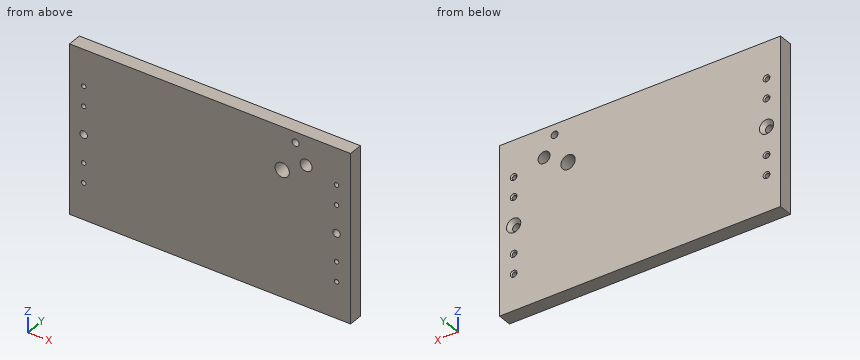
```python
from build123d import *

# Parameters (mm, degrees)
SKETCH1_W                                        = 254
SKETCH1_H                                        = 152.4
BOSS_EXTRUDE1_DEPTH                              = 12.7
SKETCH2_W                                        = 203.2
SKETCH2_H                                        = 63.5
CUT_EXTRUDE1_DEPTH                               = 149.649688866
SKETCH11_W                                       = 203.2
SKETCH11_H                                       = 63.5
BOSS_EXTRUDE2_DEPTH                              = 12.7
SKETCH13_R                                       = 5.3578125
SKETCH13_R_2                                     = 6.4897
CUT_EXTRUDE8_DEPTH                               = 149.649688866
SKETCH14_R                                       = 3.1623
CUT_EXTRUDE9_DEPTH                               = 149.649688866
F_10_32_TAPPED_HOLE2_D                           = 4.0386
F_10_32_TAPPED_HOLE2_CSINK_D                     = 6.096
F_10_32_TAPPED_HOLE2_CSINK_ANGLE                 = 90
MIRROR2_COPY_1_D                                 = 4.0386
MIRROR2_COPY_1_CSINK_D                           = 6.096
MIRROR2_COPY_1_CSINK_ANGLE                       = 90
CSK_FOR_1_4_FLAT_HEAD_MACHINE_SCREW1_D           = 6.7564
CSK_FOR_1_4_FLAT_HEAD_MACHINE_SCREW1_CSINK_D     = 12.8778
CSK_FOR_1_4_FLAT_HEAD_MACHINE_SCREW1_CSINK_ANGLE = 82


with BuildPart() as part:
    # Sketch1 → Boss-Extrude1 (new body)
    with BuildSketch(Plane(origin=(0, 0, 0), x_dir=(1, 0, 0), z_dir=(0, 1, 0))):
        Rectangle(SKETCH1_W, SKETCH1_H)
    extrude(amount=BOSS_EXTRUDE1_DEPTH)

    # Sketch2 → Cut-Extrude1 (cut, through all)
    with BuildSketch(Plane(origin=(0, 12.7, 0), x_dir=(1, 0, 0), z_dir=(0, 1, 0))):
        with Locations((0, -44.45)):
            Rectangle(SKETCH2_W, SKETCH2_H)
        with Locations((0, 44.45)):
            Rectangle(SKETCH2_W, SKETCH2_H)
    extrude(amount=-CUT_EXTRUDE1_DEPTH, mode=Mode.SUBTRACT)

    # Sketch11 → Boss-Extrude2 (add)
    with BuildSketch(Plane(origin=(0, 12.7, 0), x_dir=(1, 0, 0), z_dir=(0, 1, 0))):
        with Locations((0, 44.45)):
            Rectangle(SKETCH11_W, SKETCH11_H)
        with Locations((0, -44.45)):
            Rectangle(SKETCH11_W, SKETCH11_H)
    extrude(amount=-BOSS_EXTRUDE2_DEPTH)

    # Sketch13 → Cut-Extrude8 (cut, through all)
    with BuildSketch(Plane(origin=(0, 12.7, 0), x_dir=(1, 0, 0), z_dir=(0, 1, 0))):
        with Locations(Location((86.819046868, -50.12500008, 0), (0, 0, 270))):
            Circle(SKETCH13_R)
        with Locations(Location((65.16841174, -37.625000061, 0), (0, 0, 270))):
            Circle(SKETCH13_R_2)
    extrude(amount=-CUT_EXTRUDE8_DEPTH, mode=Mode.SUBTRACT)

    # Sketch14 → Cut-Extrude9 (cut, through all)
    with BuildSketch(Plane(origin=(0, 12.7, 0), x_dir=(1, 0, 0), z_dir=(0, 1, 0))):
        with Locations(Location((77.237896866, -66.720038678, 0), (0, 0, 270))):
            Circle(SKETCH14_R)
    extrude(amount=-CUT_EXTRUDE9_DEPTH, mode=Mode.SUBTRACT)

    # #10-32 Tapped Hole2 (through all)
    with Locations(Plane(origin=(0, 12.7, 0), x_dir=(1, 0, 0), z_dir=(0, 1, 0))):
        with Locations((-114.3, -25.3365), (-114.3, -43.2435)):
            f_10_32_tapped_hole2 = CounterSinkHole(F_10_32_TAPPED_HOLE2_D / 2, F_10_32_TAPPED_HOLE2_CSINK_D / 2, counter_sink_angle=F_10_32_TAPPED_HOLE2_CSINK_ANGLE)

    # Mirror1: #10-32 Tapped Hole2 across plane
    add(f_10_32_tapped_hole2.mirror(Plane.XY), mode=Mode.SUBTRACT)

    # Mirror2: #10-32 Tapped Hole2 across plane
    add(f_10_32_tapped_hole2.mirror(Plane(origin=(0, 0, 0), x_dir=(0, 0, 1), z_dir=(1, 0, 0))), mode=Mode.SUBTRACT)

    # Mirror2 copy 1 (through all)
    with Locations(Plane(origin=(0, 12.7, 0), x_dir=(-1, 0, 0), z_dir=(0, 1, 0))):
        with Locations((-114.3, -25.3365), (-114.3, -43.2435)):
            CounterSinkHole(MIRROR2_COPY_1_D / 2, MIRROR2_COPY_1_CSINK_D / 2, counter_sink_angle=MIRROR2_COPY_1_CSINK_ANGLE)

    # CSK for 1/4 Flat Head Machine Screw1 (through all)
    with Locations(Plane(origin=(0, 12.7, 0), x_dir=(1, 0, 0), z_dir=(0, 1, 0))):
        with Locations((-114.3, 0)):
            csk_for_1_4_flat_head_machine_screw1 = CounterSinkHole(CSK_FOR_1_4_FLAT_HEAD_MACHINE_SCREW1_D / 2, CSK_FOR_1_4_FLAT_HEAD_MACHINE_SCREW1_CSINK_D / 2, counter_sink_angle=CSK_FOR_1_4_FLAT_HEAD_MACHINE_SCREW1_CSINK_ANGLE)

    # Mirror3: CSK for 1/4 Flat Head Machine Screw1 across plane
    add(csk_for_1_4_flat_head_machine_screw1.mirror(Plane(origin=(0, 0, 0), x_dir=(0, 0, 1), z_dir=(1, 0, 0))), mode=Mode.SUBTRACT)


solid = part.part
```
CAD build for the part. Positions are in the model's coordinates, mm. Give positions to 0.01 mm unless a question says otherwise; leave off trailing zeros. Write each loop counter-clockwise with the first axis right and the second up, starting at its lowest first coordinate (ties: lowest second). Pieces come first, ordered by that corner, then holes. Notation, with made-up numbers: M 27.5,-5 L 76.5,-5 A14 cw 76.5,21 Z; hole C -37.75,54.5 d8. An arc over 180 degrees is marked long. Return JSON: item names as keys, results as strings. Group by question number.
(1) Drill centre lines: L1, parallel to X at y = 3.25, z = -1.5; L2, parallel to X at y = 0.75, z = -25.5; L3, parallel to Z at x = -114.3, y = 6. Where is each one in solid material? Low to high. Write a range as [from, to].
(2) Band-saw the part on A-A (z = 0). Give the cut face in (x, y).
(3) Flat gauge pins, fed straight in: pin 1 Ø5.5 at (x, z) = (-114.3, 43.24) entering from +Y; pin 2 Ø3.5 at (x, z) = (114.3, -25.34) entering from +Y; pin 3 Ø8 at (x, z) = (114.3, 0) entering from +Y. Where does each tip first touch, or does it go through?
Entries:
{
 "1": {"L1": "x = [-127, -117.33], [-111.27, 111.27], [117.33, 127]", "L2": "x = [-127, -116.31], [-112.29, 112.29], [116.31, 127]", "L3": "z = [-76.2, -45.26], [-41.22, -27.36], [-23.32, -3.38], [3.38, 23.32], [27.36, 41.22], [45.26, 76.2]"},
 "2": {"outline": "M -127,0 L -117.68,0 L -117.68,9.18 L -120.74,12.7 L -127,12.7 Z; M -110.92,0 L 110.92,0 L 110.92,9.18 L 107.86,12.7 L -107.86,12.7 L -110.92,9.18 Z; M 117.68,0 L 127,0 L 127,12.7 L 120.74,12.7 L 117.68,9.18 Z"},
 "3": {"pin 1": "stops at y = 12.41", "pin 2": "passes through", "pin 3": "stops at y = 9.89"}
}
